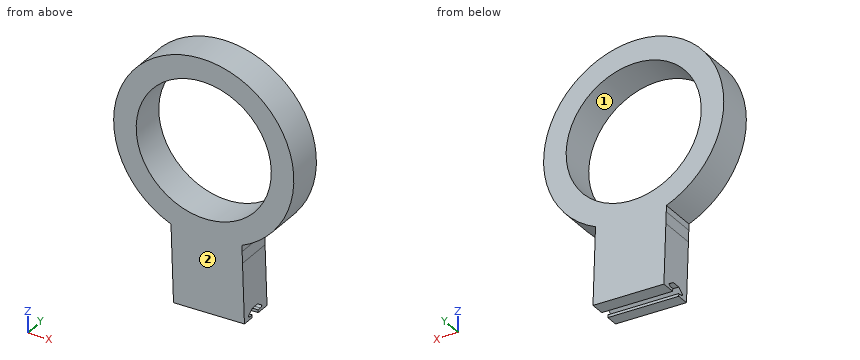
from build123d import *

# Parameters (mm, degrees)
SKETCH1_R               = 50.8
SKETCH1_R_2             = 38.1
BOSS_EXTRUDE1_DEPTH     = 20
BOSS_EXTRUDE2_START     = -20
BOSS_EXTRUDE2_DEPTH     = 20
CUT_EXTRUDE1_DEPTH      = 118.349403873
CUT_EXTRUDE1_DEPTH_BACK = 118.349403873
FILLET1_R               = 1.27


with BuildPart() as part:
    # Sketch1 → Boss-Extrude1 (new body)
    with BuildSketch(Plane(origin=(0, 0, 0), x_dir=(1, 0, 0), z_dir=(0, 1, 0))):
        with Locations(Location((0, 0, 0), (0, 0, 270))):
            Circle(SKETCH1_R)
        with Locations(Location((0, 0, 0), (0, 0, 270))):
            Circle(SKETCH1_R_2, mode=Mode.SUBTRACT)
    extrude(amount=BOSS_EXTRUDE1_DEPTH)

    # Sketch2 → Boss-Extrude2 (add)
    with BuildSketch(Plane(origin=(0, 20, 0), x_dir=(1, 0, 0), z_dir=(0, 1, 0)).offset(BOSS_EXTRUDE2_START)):
        with BuildLine():
            ThreePointArc((9.793574848, 49.847024903), (15.777570545, 48.287765197), (21.527776819, 46.012985398))
            Line((21.527776819, 46.012985398), (21.640596186, 49.459185087))
            Line((21.640596186, 49.459185087), (9.793574848, 49.847024903))
        make_face()
        with BuildLine():
            Line((-18.147499758, 57.241535713), (-18.359403814, 50.768678182))
            Line((-18.359403814, 50.768678182), (-6.512382476, 50.380838366))
            ThreePointArc((-6.512382476, 50.380838366), (1.662165771, 50.772799853), (9.793574848, 49.847024903))
            Line((9.793574848, 49.847024903), (21.640596186, 49.459185087))
            Line((21.640596186, 49.459185087), (21.852500242, 55.932042618))
            Line((21.852500242, 55.932042618), (-18.147499758, 57.241535713))
        make_face()
        with BuildLine():
            Line((-18.359403814, 50.768678182), (-18.472223181, 47.322478493))
            ThreePointArc((-18.472223181, 47.322478493), (-12.585548111, 49.216297898), (-6.512382476, 50.380838366))
            Line((-6.512382476, 50.380838366), (-18.359403814, 50.768678182))
        make_face()
        Polygon((-17.049910719, 90.768678182), (-18.147499758, 57.241535713), (21.852500242, 55.932042618), (22.950089281, 89.459185087), align=None)
    extrude(amount=BOSS_EXTRUDE2_DEPTH)

    # Sketch4 → Cut-Extrude1 (cut, two sides: drawn at the far end of the back side and taken through both)
    with BuildSketch(Plane(origin=(20, 0, 0.654746548), x_dir=(0.03271979863396448, 0, -0.9994645640428443), z_dir=(0.9994645640428443, 0, 0.03271979863396448)).offset(-CUT_EXTRUDE1_DEPTH_BACK)):
        Polygon((90.162207723, 12.222487003), (88.638207723, 12.222487003), (88.638207723, 15.524487003), (87.622207723, 15.524487003), (85.172720429, 11.968487003), (85.172720429, 7.142487003), (87.622207723, 3.586487003), (88.638207723, 3.586487003), (88.638207723, 6.888487003), (90.162207723, 6.888487003), align=None)
    extrude(amount=CUT_EXTRUDE1_DEPTH + CUT_EXTRUDE1_DEPTH_BACK, mode=Mode.SUBTRACT)

    # Fillet1
    # the kernel refuses this fillet: 1.27 mm, written as the material it adds along each edge
    with BuildSketch(Plane(origin=(-17.099775692, 3.586487003, -89.245494187), x_dir=(-0.032719798633964424, 1.5621799566964636e-12, 0.9994645640428443), z_dir=(0.9994645640428443, 0, 0.03271979863396443))) as fillet1_piece_1:
        with BuildLine():
            CenterArc((1.27, -1.244340789), FILLET1_R, 101.536959033, 78.463040967)
            Line((0, -1.244340789), (-0.0254, -1.244340789))
            Line((-0.0254, -1.244340789), (-0.0254, 0))
            Line((-0.0254, 0), (0, 0.0254))
            ThreePointArc((0, 0.0254), (0.508, 0.0254), (1.01092, 0.024886816))
            Line((1.01092, 0.024886816), (1.016, 0))
        make_face()
    extrude(amount=40.021428912)
    with BuildSketch(Plane(origin=(-17.099775692, 15.524487003, -89.245494187), x_dir=(0, -1, 0), z_dir=(0.9994645640428443, 0, 0.03271979863396443))) as fillet1_piece_2:
        with BuildLine():
            CenterArc((1.244340789, -1.27), FILLET1_R, 90, 78.463040967)
            Line((0, -1.016), (-0.024886816, -1.01092))
            ThreePointArc((-0.024886816, -1.01092), (-0.0254, -0.508), (-0.0254, 0))
            Line((-0.0254, 0), (0, 0.0254))
            Line((0, 0.0254), (1.244340789, 0.0254))
            Line((1.244340789, 0.0254), (1.244340789, 0))
        make_face()
    extrude(amount=40.021428912)


solid = part.part
Can you work these out from the model? Positions are in its coordinate system, mm. Face numbers are marked on the shaded views. Round coordinates to 2 decimals unless told otherwise and drop trailing zeros. Order: outer loops, then holes, each group sorted by start corner. A loop starts at its lowest first (then second) coordinate and runs counter-clockwise, first axis right, second up. Notation, with made-up numbers: (44, 10) - (72, 10) arc R18 cw to (72, 39) - close; hole circle Ø2 at (88, 45). An arc over 180 degrees is marked (long way). Answer in a Markdown table with one row per item.
(1) Suppose I cut it at D-D, the plane z = -63.5. Please give me the cut outline in (x, y), plus the area to 3 significant figures.
From the geometry:
| item | result |
|---|---|
| outline | (-17.94, 0) - (22.1, 0) - (22.1, 20) - (-17.94, 20) - close |
| area | 801 mm2 |
(2) Please list where these lines run through material, in increasing order: L1, parallel to X at y = 14, z = 0; L2, parallel to Z at x = -33, y = 18.25; L3, parallel to Z at x = -2, y = 6. Write a range as from..to.
From the geometry:
| item | result |
|---|---|
| L1 | x = -50.8..-38.1, 38.1..50.8 |
| L2 | z = -38.62..-19.04, 19.04..38.62 |
| L3 | z = -90.28..-88.75, -86.07..-38.05, 38.05..50.76 |
(3) For P1, Ø2, axis at x = -31.5, z = -20.5, coming from the -Y side; P2, Ø4, axis at x = -29.5, y = 13.5, coming from the +Z side; P3, Ø10, axis at y = 2.5, z = -46, coming from the +X side; P4, Ø5, axis at y = 16, z = -29, coming from the +X side, each with a flat end and sliding along its axis, tell me the tip position at first contact or that it passes through.
From the geometry:
| item | result |
|---|---|
| P1 | stops at y = 0 |
| P2 | stops at z = 42.71 |
| P3 | stops at x = 29.99 |
| P4 | stops at x = 43.34 |
(4) Suppose I cut it at C-C, the plane x = -32.5. Please give me the cut outline in (y, z).
From the geometry:
| item | result |
|---|---|
| outline | (0, -39.04) - (20, -39.04) - (20, -19.88) - (0, -19.88) - close; (0, 19.88) - (20, 19.88) - (20, 39.04) - (0, 39.04) - close |
(5) Suppose I cut it at A-A, the plane z = 0. Please give me the cut outline in (x, y), plus the area to 3 significant figures.
From the geometry:
| item | result |
|---|---|
| outline | (-50.8, 0) - (-38.1, 0) - (-38.1, 20) - (-50.8, 20) - close; (38.1, 0) - (50.8, 0) - (50.8, 20) - (38.1, 20) - close |
| area | 508 mm2 |
(6) If we mould it in two halves opening along Z, with no side actions, what happens to the marked faces 1 and 2? For each: released by +Z, released by -Z, zero draft, split by the parting line, or undercut.
From the geometry:
| item | result |
|---|---|
| face 1 | undercut |
| face 2 | zero draft |
(7) Suppose I cut it at B-B, the plane y = 1.75. Please give me the cut outline in (x, z).
From the geometry:
| item | result |
|---|---|
| outline | (-18.47, -47.32) - (-17.05, -90.77) - (22.95, -89.46) - (21.53, -46.01) arc R50.8 ccw (long way) to start; hole circle Ø76.2 at (0, 0) |
